Read the model definition and answer for the solid it produces. Units are mm, in the model's axes. Face numbers are marked on the shaded views. A direction names the side the tool comes from. Give positions to 0.01 mm unless a question says otherwise; leave off trailing zeros. Loops run counter-clockwise (first coordinate to the right, second up) from the corner with the lowest first, then second, coordinate; pieces in that order, holes last. Notation, with made-up numbers: (2.25, -29) - (31.25, -29) arc R23 cw to (31.25, -3) - close; hole circle Ø6 at (23.5, 11). An arc over 180 degrees is marked (long way). Put each result on its own line as item: value. Start each with the question number.
1. Given pin 1 Ø3 at (y, z) = (12, -4) entering from -X; pin 2 Ø10 at (x, z) = (-34, -26.5) entering from +Y; pin 3 Ø3 at (y, z) = (8, 9.5) entering from +X; pin 4 Ø0.6 at (y, z) = (12.5, 31) entering from -X, each flat-ended and moving along its own axis, determine where each tip first touches the part or whether it passes through.
2. A cutting plane is placed at B-B, the plane z = -25. Determine the outline of the cut face in (x, y).
3. Consider L1, parallel to Z at x = 21.5, y = 10.5; L2, parallel to X at y = 6.75, z = 25; L3, parallel to Y at x = 20, z = 31.5. Determine where each line is inside the solid, lowest interval first. Write a range as from..to.
4. A cutting plane is placed at C-C, the plane x = 12. Determine the outline of the cut face in (y, z), plus the area to 3 significant figures.
5. A cutting plane is placed at A-A, the plane y = 8.25. Determine the outline of the cut face in (x, z), plus the area to 3 significant figures.
6. For a pull along X with two mould halves and no side action, classify the marked faces 3, 4 and 5 as released by +X, released by -X, zero draft, split by the parting line, or undercut.
7. For the marked faces 1 and 2, determine the directions among +Z, -Z, +X, -X, +Y, -Y from which every point of the face is accessible in a straight line to the end or side of a thin tool.
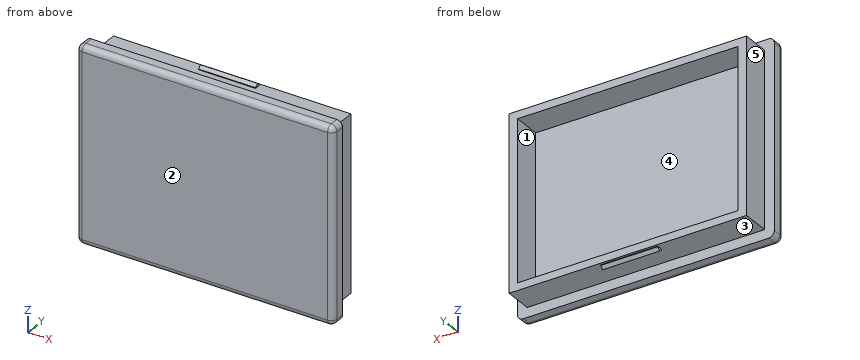
Autodesk Fusion 360 part; units mm, degrees
sketch "Sketch1" plane through (0, 0, 0) normal (0, 1, 0) x (1, 0, 0)
  line L0 (47, 36) -> (-47, 36)
  line L1 (-47, 36) -> (-47, -36)
  line L2 (-47, -36) -> (47, -36)
  line L3 (47, -36) -> (47, 36)
  line L4 (47, 36) -> (-47, -36) construction
  line L5 (-47, 36) -> (47, -36) construction
  dimension "d1" = 72
  dimension "d2" = 94
extrude "Extrude1" add sketch "Sketch1" along normal blind 5
sketch "Sketch2" plane through (0, 5, 0) normal (0, 1, 0) x (-1, 0, 0)
  line L0 (-47, 36) -> (-47, -36)
  line L1 (-47, -36) -> (47, -36)
  line L2 (47, -36) -> (47, 36)
  line L3 (47, 36) -> (-47, 36)
  line L4 (-41.6, -30.6) -> (41.6, -30.6)
  line L5 (41.6, -30.6) -> (41.6, 30.6)
  line L6 (41.6, 30.6) -> (-41.6, 30.6)
  line L7 (-41.6, 30.6) -> (-41.6, -30.6)
  line L8 (-41.6, -30.6) -> (41.6, 30.6) construction
  line L9 (41.6, -30.6) -> (-41.6, 30.6) construction
  dimension "d5" = 83.2
  dimension "d6" = 61.2
extrude "Extrude2" add sketch "Sketch2" along normal blind 9.8 contours L4 L5 L6 L7
fillet "Fillet1" radius 2 4 edges at (47, 2.5, -36) (47, 2.5, 36) (-47, 2.5, 36) (-47, 2.5, -36)
fillet "Fillet2" radius 2 8 edges at (0, 0, -36) (-46.4142, 0, -35.4142) (-47, 0, 0) (-46.4142, 0, 35.4142) (0, 0, 36) (46.4142, 0, 35.4142) (47, 0, 0) (46.4142, 0, -35.4142)
sketch "Sketch3" plane through (0, 14.8, 0) normal (0, 1, 0) x (-1, 0, 0)
  line L0 (-41.6, 30.6) -> (-41.6, -30.6)
  line L1 (-41.6, -30.6) -> (41.6, -30.6)
  line L2 (41.6, -30.6) -> (41.6, 30.6)
  line L3 (41.6, 30.6) -> (-41.6, 30.6)
  line L4 (-38.6, -28) -> (38.6, -28)
  line L5 (38.6, -28) -> (38.6, 28)
  line L6 (38.6, 28) -> (-38.6, 28)
  line L7 (-38.6, 28) -> (-38.6, -28)
  line L8 (-38.6, -28) -> (38.6, 28) construction
  line L9 (38.6, -28) -> (-38.6, 28) construction
  line L10 (-45, -34) -> (45, -34)
  dimension "d11" = 56
  dimension "d12" = 77.2
  dimension "d13" = 90
extrude "Extrude3" cut sketch "Sketch3" against normal blind 9.8 contours L4 L5 L6 L7
sketch "Sketch4" plane through (0, 0, -30.6) normal (0, 0, -1) x (-1, 0, 0)
  line L0 (-41.6, 5) -> (41.6, 5)
  line L1 (41.6, 5) -> (41.6, 14.8)
  line L2 (41.6, 14.8) -> (-41.6, 14.8)
  line L3 (-41.6, 14.8) -> (-41.6, 5)
  line L4 (10, 14) -> (-10, 14)
  line L5 (-10, 14) -> (-10, 12)
  line L6 (-10, 12) -> (10, 12)
  line L7 (10, 12) -> (10, 14)
  line L8 (10, 14) -> (-10, 12) construction
  line L9 (-10, 14) -> (10, 12) construction
  point P0 (0, 13)
  dimension "d16" = 20
  dimension "d17" = 2
extrude "Extrude4" add sketch "Sketch4" along normal blind 1.2 contours L4 L5 L6 L7
sketch "Sketch5" plane through (10, 0, 0) normal (1, 0, 0) x (0, 0, -1)
  line L0 (30.6, 14) -> (30.6, 12)
  line L1 (30.6, 12) -> (31.8, 12)
  line L2 (31.8, 12) -> (31.8, 14)
  line L3 (31.8, 14) -> (30.6, 14)
  point P0 (31.8, 14)
  point P1 (31.8, 12)
  point P2 (31.8, 12)
  point P3 (31.8, 12)
  point P4 (31.8, 12)
  point P5 (31.8, 12)
  point P6 (31.8, 14)
  point P7 (31.8, 14)
  point P8 (31.8, 14)
  point P9 (31.8, 14)
  point P10 (31.8, 14)
  point P11 (31.8, 14)
  point P12 (31.8, 14)
  point P13 (31.8, 14)
  point P14 (31.8, 14)
  point P15 (31.8, 14)
  point P16 (31.8, 12)
  point P17 (31.8, 14)
  point P18 (31.8, 12)
  point P19 (31.8, 14)
ref_plane "WorkPlane2" through (0, 9.9, 0) normal (0, 0, 1) x (-1, 0, 0)
ref_plane "WorkPlane1" through (0, 9.9, 30.6) normal (0, 0, 1) x (1, 0, 0)
ref_plane "WorkPlane3" through (0, 13, -26.8) normal (0, 0, -1) x (-1, 0, 0)
ref_plane "WorkPlane4" through (0, 13, -26.8) normal (0, 0, -1) x (-1, 0, 0)
mirror "Mirror1" about plane through (0, 9.9, 0) normal (0, 0, 1) of "Extrude4"
chamfer "Chamfer1" distance 1 angle 45 2 edges at (0, 14, 31.8) (0, 12, 31.8)
chamfer "Chamfer2" distance 1 angle 45 2 edges at (0, 14, -31.8) (0, 12, -31.8)
sketch "Sketch6" plane through (0, 14.8, 0) normal (0, 1, 0) x (-1, 0, 0)
  line L0 (38.6, -28) -> (-38.6, -28)
  line L1 (-38.6, -28) -> (-38.6, 28)
  line L2 (-38.6, 28) -> (38.6, 28)
  line L3 (38.6, 28) -> (38.6, -28)
  line L4 (-41.6, 30.6) -> (-41.6, -30.6)
  line L5 (-41.6, -30.6) -> (41.6, -30.6)
  line L6 (41.6, -30.6) -> (41.6, 30.6)
  line L7 (41.6, 30.6) -> (-41.6, 30.6)
  point P0 (42.1144, 28)
  point P1 (-41.6, 30.6)
sketch "Sketch7" plane through (0, 5, 0) normal (0, 1, 0) x (-1, 0, 0)
  arc A0 (45, -36) -> (47, -34) centre (45, -34) ccw
  line L0 (47, -34) -> (47, 34)
  arc A1 (47, 34) -> (45, 36) centre (45, 34) ccw
  line L1 (45, 36) -> (-45, 36)
  arc A2 (-45, 36) -> (-47, 34) centre (-45, 34) ccw
  line L2 (-47, 34) -> (-47, -34)
  arc A3 (-47, -34) -> (-45, -36) centre (-45, -34) ccw
  line L3 (-45, -36) -> (45, -36)
  line L4 (-41.6, 30.6) -> (41.6, 30.6)
  line L5 (41.6, 30.6) -> (41.6, -30.6)
  line L6 (41.6, -30.6) -> (-41.6, -30.6)
  line L7 (-41.6, -30.6) -> (-41.6, 30.6)
  line L8 (45, -34) -> (-45, -34)
  line L9 (-45, -34) -> (-45, 34)
  line L10 (-45, 34) -> (45, 34)
  line L11 (45, 34) -> (45, -34)
extrude "Extrude5" cut sketch "Sketch7" against normal blind 5 contours A0 L0 A1 L1 A2 L2 A3 L3
fillet "Fillet3" radius 2 8 edges at (-45, 2.5, -34) (0, 0, -34) (-45, 0, 0) (45, 2.5, -34) (45, 0, 0) (45, 2.5, 34) (0, 0, 34) (-45, 2.5, 34)
Return value:
1. pin 1: stops at x = -41.6
1. pin 2: stops at y = 14.8
1. pin 3: stops at x = 41.6
1. pin 4: stops at x = -10
2. outline: (-45, 2) arc R2 ccw to (-43, 0) - (43, 0) arc R2 ccw to (45, 2) - (45, 5) - (41.6, 5) - (41.6, 14.8) - (38.6, 14.8) - (38.6, 5) - (-38.6, 5) - (-38.6, 14.8) - (-41.6, 14.8) - (-41.6, 5) - (-45, 5) - close
3. L1: z = -30.6..-28, 28..30.6
3. L2: x = -41.6..-38.6, 38.6..41.6
3. L3: y = 0..5
4. outline: (0, -32) arc R2 ccw to (2, -34) - (5, -34) - (5, -30.6) - (14.8, -30.6) - (14.8, -28) - (5, -28) - (5, 28) - (14.8, 28) - (14.8, 30.6) - (5, 30.6) - (5, 34) - (2, 34) arc R2 ccw to (0, 32) - close
4. area: 389 mm2
5. outline: (-41.6, -30.6) - (41.6, -30.6) - (41.6, 30.6) - (-41.6, 30.6) - close; hole (-38.6, -28) - (38.6, -28) - (38.6, 28) - (-38.6, 28) - close
5. area: 769 mm2
6. face 3: zero draft
6. face 4: undercut
6. face 5: released by -X
7. face 1: +Y
7. face 2: +Z, -Z, +X, -X, -Y
